Read the model definition and answer for the solid it produces. Units are mm, in the model's axes. A direction names the side the tool comes from. Coordinates: 2 decimals unless noted, no trailing zeros. Loops run counter-clockwise (first coordinate to the right, second up) from the corner with the lowest first, then second, coordinate; pieces in that order, holes last. Notation, with made-up numbers: (-25, 11) - (0, 11) arc R24 cw to (0, 25) - close; hole circle Ø8 at (51, 2). An arc over 180 degrees is marked (long way). Use one line per item in the form item = value.
from build123d import *

# Parameters (mm, degrees)
SKETCH1_R           = 1.5
BOSS_EXTRUDE1_DEPTH = 3
BOSS_EXTRUDE2_DEPTH = 25
SKETCH6_W           = 56
SKETCH6_H           = 9.11547301
CUT_EXTRUDE1_DEPTH  = 63.91555103
FILLET1_R           = 2
FILLET2_R           = 1


with BuildPart() as part:
    # Sketch1 → Boss-Extrude1 (new body)
    with BuildSketch(Plane.XY):
        with BuildLine():
            Line((-3.762452186, -3.055345405), (1.803522753, -8.621320344))
            ThreePointArc((1.803522753, -8.621320344), (2.453841007, -9.59459039), (2.68220241, -10.742640687))
            Line((2.68220241, -10.742640687), (2.68220241, -18.5))
            ThreePointArc((2.68220241, -18.5), (2.975095629, -19.207106781), (3.68220241, -19.5))
            Line((3.68220241, -19.5), (18.54616344, -19.5))
            ThreePointArc((18.54616344, -19.5), (19.008103207, -19.191341716), (18.899716831, -18.646446609))
            Line((18.899716831, -18.646446609), (2.601508845, -2.348238623))
            ThreePointArc((2.601508845, -2.348238623), (2.308615626, -1.641131842), (2.601508845, -0.934025061))
            Line((2.601508845, -0.934025061), (2.927422074, -0.608111832))
            ThreePointArc((2.927422074, -0.608111832), (3.220315293, 0.098994949), (2.927422074, 0.806101731))
            Line((2.927422074, 0.806101731), (0.806101731, 2.927422074))
            ThreePointArc((0.806101731, 2.927422074), (0.098994949, 3.220315293), (-0.608111832, 2.927422074))
            Line((-0.608111832, 2.927422074), (-1.641131842, 1.894402064))
            Line((-1.641131842, 1.894402064), (-3.762452186, -0.22691828))
            ThreePointArc((-3.762452186, -0.22691828), (-4.348238623, -1.641131842), (-3.762452186, -3.055345405))
        make_face()
        Circle(SKETCH1_R, mode=Mode.SUBTRACT)
    boss_extrude1 = extrude(amount=BOSS_EXTRUDE1_DEPTH)

    # Sketch2 → Boss-Extrude2 (add)
    with BuildSketch(Plane.XY.offset(3)):
        with BuildLine():
            Line((18.899716831, -18.646446609), (10.995910909, -10.742640687))
            Line((10.995910909, -10.742640687), (2.68220241, -10.742640687))
            Line((2.68220241, -10.742640687), (2.68220241, -18.5))
            ThreePointArc((2.68220241, -18.5), (2.975095629, -19.207106781), (3.68220241, -19.5))
            Line((3.68220241, -19.5), (18.54616344, -19.5))
            ThreePointArc((18.54616344, -19.5), (19.008103207, -19.191341716), (18.899716831, -18.646446609))
        make_face()
    boss_extrude2 = extrude(amount=BOSS_EXTRUDE2_DEPTH)

    # Mirror1: Boss-Extrude1, Boss-Extrude2 across plane
    add(boss_extrude1.mirror(Plane.XY.offset(28)))
    add(boss_extrude2.mirror(Plane.XY.offset(28)))

    # Sketch6 → Cut-Extrude1 (cut, through all)
    with BuildSketch(Plane(origin=(-6.530219139, -6.530219139, 0), x_dir=(0, 0, 1), z_dir=(-0.7071067811865487, -0.7071067811865465, 0))):
        with Locations((28, -17.586068001)):
            Rectangle(SKETCH6_W, SKETCH6_H)
    extrude(amount=CUT_EXTRUDE1_DEPTH, mode=Mode.SUBTRACT)

    # Fillet1
    fillet1_edges = [part.edges().sort_by_distance(p)[0] for p in [
        (6.439561723, -19.5, 28),
    ]]
    fillet(fillet1_edges, radius=FILLET1_R)

    # Fillet2
    fillet2_edges = [part.edges().sort_by_distance(p)[0] for p in [
        (2.68220241, -15.742640687, 28),
    ]]
    fillet(fillet2_edges, radius=FILLET2_R)


solid = part.part
Item 1: Which of the six approach directions +Z, -Z, +X, -X, +Y, -Y give full straight-line access (tool end or side, diameter ignored) to faces 1 (the cylindrical face through (-4.35, -1.62, 54.52)), 2 (the flat face through (7, -10.743, 28))?
Results below:
face_1 = +Z, -Z, -X
face_2 = +X, -X, +Y
Item 2: Find the intervals of material crossed by L1, parallel to Z at x = 7.5, y = -7.5; L2, parallel to Y at x = 0, z = 54.45; L3, parallel to Y at x = 16.25, z = 15, in increasing order.
Results below:
L1 = 0 to 3, 53 to 56
L2 = -6.82 to -1.5, 1.5 to 3.22
L3 = -19.5 to -16
Item 3: For a pull along Y with two mould halves and no side action, classify faces 3 (the cylindrical face through (6.51, -19.35, 27.61)), 4 (the flat face through (-2.163, 1.372, 54.521)), 5 (the flat face through (2.682, -13, 28)), 6 (the cylindrical face through (2.31, -1.65, 54.52)) as +Y half, -Y half, draft (parallel to the pull), parting line (faces both ways), or undercut.
Results below:
face_3 = -Y half
face_4 = +Y half
face_5 = draft
face_6 = undercut
Item 4: Each of these flat-tipped pins is pushed along its axis until it touches: P1, Ø5, axis at x = 0, y = 0, coming from the -Z side; P2, Ø5, axis at x = 5, z = 47.5, coming from the +Y side; P3, Ø12, axis at y = -7, z = 34.5, coming from the +X side; P4, Ø1.8, axis at x = 0, y = 0, coming from the -Z side. Where does it stop, or does it pass through?
Results below:
P1 = 0
P2 = -10.74
P3 = 13.25
P4 = through
Item 5: The part is cut by section A-A on z = 14. Give the vertices of the cut face in (x, y).
Results below:
outline = (2.68, -15.33) arc R1 ccw to (2.98, -16.04) - (5.85, -18.91) arc R2 ccw to (7.27, -19.5) - (18.55, -19.5) arc R0.5 ccw to (18.9, -18.65) - (11, -10.74) - (2.68, -10.74) - close
Item 6: The part is cut by section D-D on x = -2.5. Give the vertices of the cut face in (y, z).
Results below:
outline = (-4.32, 0) - (1.04, 0) - (1.04, 3) - (-4.32, 3) - close; (-4.32, 53) - (1.04, 53) - (1.04, 56) - (-4.32, 56) - close
Item 7: The part is cut by section C-C on y = -4.5. Give the vertices of the cut face in (x, z), plus the area to 3 significant figures.
Results below:
outline = (-2.32, 0) - (4.75, 0) - (4.75, 3) - (-2.32, 3) - close; (-2.32, 53) - (4.75, 53) - (4.75, 56) - (-2.32, 56) - close
area = 42.4 mm²
Item 8: The part is cut by section B-B on x = 0. Give the vertices of the cut face in (y, z).
Results below:
outline = (-6.82, 0) - (-1.5, 0) - (-1.5, 3) - (-6.82, 3) - close; (-6.82, 53) - (-1.5, 53) - (-1.5, 56) - (-6.82, 56) - close; (1.5, 0) - (3.22, 0) - (3.22, 3) - (1.5, 3) - close; (1.5, 53) - (3.22, 53) - (3.22, 56) - (1.5, 56) - close
